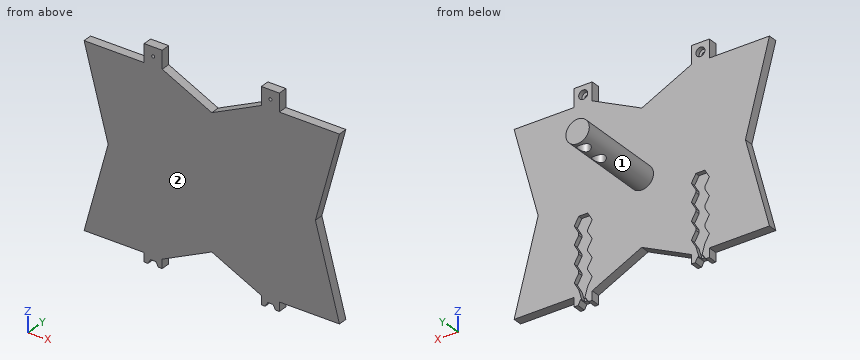
from build123d import *

# Parameters (mm, degrees)
CROQUIS1_R              = 0.5
SALIENTE_EXTRUIR1_DEPTH = 3
CROQUIS2_R              = 3.9
SALIENTE_EXTRUIR2_DEPTH = 30
CROQUIS3_R              = 2
CORTAR_EXTRUIR1_DEPTH   = 64
CROQUIS4_R              = 1.5
CORTAR_EXTRUIR2_DEPTH   = 1.5
CORTAR_EXTRUIR3_DEPTH   = 1.5


with BuildPart() as part:
    # Croquis1 → Saliente-Extruir1 (new body)
    with BuildSketch(Plane(origin=(0, 0, 0), x_dir=(1, 0, 0), z_dir=(0, 1, 0))):
        Polygon((30, 60), (30, 63), (31.267949192, 63), (32.133974596, 61.5), (33.866025404, 61.5), (34.732050808, 63), (36, 63), (36, 60), (52.5, 52), (69, 60), (69, 63), (70.267949192, 63), (71.133974596, 61.5), (72.866025404, 61.5), (73.732050808, 63), (75, 63), (75, 60), (95, 60), (87, 30), (95, 0), (75, 0), (75, -6), (69, -6), (69, 0), (52.5, 8), (36, 0), (36, -6), (30, -6), (30, 0), (10, 0), (18, 30), (10, 60), align=None)
        with Locations((33, -3)):
            Circle(CROQUIS1_R, mode=Mode.SUBTRACT)
        with Locations((72, -3)):
            Circle(CROQUIS1_R, mode=Mode.SUBTRACT)
    extrude(amount=SALIENTE_EXTRUIR1_DEPTH)

    # Croquis2 → Saliente-Extruir2 (add)
    with BuildSketch(Plane(origin=(0, 3, 0), x_dir=(1, 0, 0), z_dir=(0, 1, 0))):
        with Locations((52.5, 30)):
            Circle(CROQUIS2_R)
    extrude(amount=SALIENTE_EXTRUIR2_DEPTH)

    # Croquis3 → Cortar-Extruir1 (cut, through all)
    with BuildSketch(Plane.XY):
        with Locations((52.5, 30)):
            Circle(CROQUIS3_R)
        with Locations((52.5, 23)):
            Circle(CROQUIS3_R)
    extrude(amount=-CORTAR_EXTRUIR1_DEPTH, mode=Mode.SUBTRACT)

    # Croquis4 → Cortar-Extruir2 (cut)
    with BuildSketch(Plane(origin=(0, 3, 0), x_dir=(1, 0, 0), z_dir=(0, 1, 0))):
        with Locations((33, -3)):
            Circle(CROQUIS4_R)
        with Locations((72, -3)):
            Circle(CROQUIS4_R)
    extrude(amount=-CORTAR_EXTRUIR2_DEPTH, mode=Mode.SUBTRACT)

    # Croquis5 → Cortar-Extruir3 (cut)
    with BuildSketch(Plane(origin=(0, 3, 0), x_dir=(1, 0, 0), z_dir=(0, 1, 0))):
        Polygon((32.5, 61.5), (33.5, 61.5), (34.5, 58.098076211), (36, 55.5), (34.5, 52.901923789), (34.5, 52.098076211), (36, 49.5), (34.5, 46.901923789), (34.5, 46.098076211), (36, 43.5), (34.5, 40.901923789), (34.5, 40.098076211), (36, 37.5), (34.5, 34.901923789), (31.5, 34.901923789), (30, 37.5), (31.5, 40.098076211), (31.5, 40.901923789), (30, 43.5), (31.5, 46.098076211), (31.5, 46.901923789), (30, 49.5), (31.5, 52.098076211), (31.5, 52.901923789), (30, 55.5), (31.5, 58.098076211), align=None)
        Polygon((71.5, 61.5), (70.5, 58.098076211), (69, 55.5), (70.5, 52.901923789), (70.5, 52.098076211), (69, 49.5), (70.5, 46.901923789), (70.5, 46.098076211), (69, 43.5), (70.5, 40.901923789), (70.5, 40.098076211), (69, 37.5), (70.5, 34.901923789), (73.5, 34.901923789), (75, 37.5), (73.5, 40.098076211), (73.5, 40.901923789), (75, 43.5), (73.5, 46.098076211), (73.5, 46.901923789), (75, 49.5), (73.5, 52.098076211), (73.5, 52.901923789), (75, 55.5), (73.5, 58.098076211), (72.5, 61.5), align=None)
    extrude(amount=-CORTAR_EXTRUIR3_DEPTH, mode=Mode.SUBTRACT)


solid = part.part
Work out the finished part from the listing and answer in its coordinate system (mm). Face numbers are marked on the shaded views. A direction names the side the tool comes from. Round coordinates to 2 decimals unless told otherwise and drop trailing zeros. Order: outer loops, then holes, each group sorted by start corner. A loop starts at its lowest first (then second) coordinate and runs counter-clockwise, first axis right, second up. Notation, with made-up numbers: M 42.25,75 L 74.25,75 A17 ccw 74.25,103 Z; hole C -11.75,-27.5 d4. An arc over 180 degrees is marked long. Put each result on its own line as item: value. Start each with the question number.
Q1. Section D-D, the plane z = -44.5 is taken. Write down the section's boundary in (x, y), and give its area (3 significant figures).
Q2. Section A-A, the plane z = -57 is taken. Write down the section's boundary in (x, y).
Q3. A tool of negligible diameter and unlimited length cuts with its end or side. For the marked faces 1 and 2, from which of +Z, -Z, +X, -X, +Y, -Y can it reach the whole face along a straight path? Write none if from no direction.
Q4. Section C-C, the plane x = 85.5 is taken. Write down the section's boundary in (y, z).
Q5. Flat-ended cylindrical pins translate along their axes: pin 1 (0.9 mm diameter, centred on x = 72.5, z = 3.5, fed in from +Y); pin 2 (0.6 mm diameter, centred on y = 2.5, z = -46.5, fed in from +X); pin 3 (8 mm diameter, centred on x = 62, y = 21, fed in from -Z); pin 4 (1.5 mm diameter, centred on y = 1, z = -61.5, fed in from -X). Find the tip coordinate at first contact, or state that the pin passes through.
Q6. Straight lines are drawn through the part: L1, parallel to X at y = 2.35, z = 3; L2, parallel to Z at x = 33, y = 1.95; L3, parallel to Z at x = 72, y = 1. For each, find the intervals that lie inside material, in ascending order. Write a range as [from, to].
Q7. Section B-B, the plane y = 24 is taken. Write down the section's boundary in (x, z), and give its area (3 significant figures).
Findings below:
1. outline: M 14.13,0 L 90.87,0 L 90.87,3 L 74.42,3 L 74.42,1.5 L 69.58,1.5 L 69.58,3 L 35.42,3 L 35.42,1.5 L 30.58,1.5 L 30.58,3 L 14.13,3 Z
1. area: 216 mm^2
2. outline: M 10.8,0 L 42.19,0 L 42.19,3 L 35.13,3 L 35.13,1.5 L 30.87,1.5 L 30.87,3 L 10.8,3 Z; M 62.81,0 L 94.2,0 L 94.2,3 L 74.13,3 L 74.13,1.5 L 69.87,1.5 L 69.87,3 L 62.81,3 Z
3. face 1: +Y
3. face 2: +Z, -Z, +X, -X, -Y
4. outline: M 0,-60 L 3,-60 L 3,0 L 0,0 Z
5. pin 1: stops at y = 1.5
5. pin 2: stops at x = 91.48
5. pin 3: passes through
5. pin 4: stops at x = 30
6. L1: x = [30, 31.5], [34.5, 36], [69, 70.5], [73.5, 75]
6. L2: z = [-34.9, 1.5], [4.5, 6]
6. L3: z = [-61.5, 2.5], [3.5, 6]
7. outline: M 50.77,-33.49 L 50.77,-26.51 A3.9 ccw Z; M 54.23,-33.49 A3.9 ccw 54.23,-26.51 Z
7. area: 21.7 mm^2
